Design review of the part built by this model. Coordinates are the model's own, in mm. A direction names the side the tool comes from. Give positions to 0.01 mm unless a question says otherwise; leave off trailing zeros. Loops run counter-clockwise (first coordinate to the right, second up) from the corner with the lowest first, then second, coordinate; pieces in that order, holes last. Notation, with made-up numbers: (58.5, 3.5) - (65.5, 3.5) arc R30 cw to (65.5, 33.5) - close; hole circle Ø10 at (33.25, 44). An arc over 180 degrees is marked (long way). Write each question's results on one line, items separated by ' | '.
```python
from build123d import *

# Parameters (mm, degrees)
SKETCH1_W           = 11
SKETCH1_H           = 12
BOSS_EXTRUDE1_DEPTH = 1.8
SKETCH2_W           = 2.54
SKETCH2_H           = 10.16
BOSS_EXTRUDE2_DEPTH = 2.54
BOSS_EXTRUDE3_START = -5.84
SKETCH3_W           = 0.5
SKETCH3_H           = 0.5
BOSS_EXTRUDE3_DEPTH = 12.34
SKETCH4_W           = 5.5
SKETCH4_H           = 4
BOSS_EXTRUDE4_DEPTH = 2
CHAMFER1_SIZE       = 0.5
SKETCH5_W           = 0.8
SKETCH5_H           = 7
BOSS_EXTRUDE5_DEPTH = 0.4
SKETCH6_R           = 0.5
CUT_EXTRUDE1_DEPTH  = 0.1
SKETCH7_R           = 0.25
CUT_EXTRUDE2_DEPTH  = 0.1


with BuildPart() as part:
    # Sketch1 → Boss-Extrude1 (new body)
    with BuildSketch(Plane(origin=(0, 0, 0), x_dir=(1, 0, 0), z_dir=(0, 1, 0))):
        Rectangle(SKETCH1_W, SKETCH1_H)
    extrude(amount=BOSS_EXTRUDE1_DEPTH)

    # Sketch2 → Boss-Extrude2 (add)
    with BuildSketch(Plane.XZ):
        with Locations((-3.81, 0)):
            Rectangle(SKETCH2_W, SKETCH2_H)
        with Locations((3.81, 0)):
            Rectangle(SKETCH2_W, SKETCH2_H)
    extrude(amount=BOSS_EXTRUDE2_DEPTH)

    # Sketch3 → Boss-Extrude3 (add)
    with BuildSketch(Plane.XZ.offset(2.54).offset(BOSS_EXTRUDE3_START)):
        with Locations((3.81, 1.27)):
            Rectangle(SKETCH3_W, SKETCH3_H)
        with Locations((3.81, 3.81)):
            Rectangle(SKETCH3_W, SKETCH3_H)
        with Locations((3.81, -1.27)):
            Rectangle(SKETCH3_W, SKETCH3_H)
        with Locations((3.81, -3.81)):
            Rectangle(SKETCH3_W, SKETCH3_H)
    boss_extrude3 = extrude(amount=BOSS_EXTRUDE3_DEPTH)

    # Mirror1: Boss-Extrude3 across plane
    add(boss_extrude3.mirror(Plane(origin=(0, 0, 0), x_dir=(0, 0, 1), z_dir=(1, 0, 0))))

    # Sketch4 → Boss-Extrude4 (add)
    with BuildSketch(Plane(origin=(0, 1.8, 0), x_dir=(1, 0, 0), z_dir=(0, 1, 0))):
        Rectangle(SKETCH4_W, SKETCH4_H)
    extrude(amount=BOSS_EXTRUDE4_DEPTH)

    # Chamfer1
    chamfer1_edges = [part.edges().sort_by_distance(p)[0] for p in [
        (0, 3.8, -2),
        (0, 3.8, 2),
    ]]
    chamfer(chamfer1_edges, length=CHAMFER1_SIZE)

    # Sketch5 → Boss-Extrude5 (add)
    with BuildSketch(Plane(origin=(0, 1.8, 0), x_dir=(1, 0, 0), z_dir=(0, 1, 0))):
        with Locations((-0.635, 0)):
            Rectangle(SKETCH5_W, SKETCH5_H)
        with Locations((-1.905, 0)):
            Rectangle(SKETCH5_W, SKETCH5_H)
        with Locations((0.635, 0)):
            Rectangle(SKETCH5_W, SKETCH5_H)
        with Locations((1.905, 0)):
            Rectangle(SKETCH5_W, SKETCH5_H)
    extrude(amount=BOSS_EXTRUDE5_DEPTH)

    # Sketch6 → Cut-Extrude1 (cut)
    with BuildSketch(Plane(origin=(0, 1.8, 0), x_dir=(1, 0, 0), z_dir=(0, 1, 0))):
        with Locations(Location((-3.81, 5.03, 0), (0, 0, 270))):
            Circle(SKETCH6_R)
    extrude(amount=-CUT_EXTRUDE1_DEPTH, mode=Mode.SUBTRACT)

    # Sketch7 → Cut-Extrude2 (cut)
    with BuildSketch(Plane(origin=(0, 3.8, 0), x_dir=(1, 0, 0), z_dir=(0, 1, 0))):
        with Locations(Location((-2.25, -1, 0), (0, 0, 270))):
            Circle(SKETCH7_R)
    extrude(amount=-CUT_EXTRUDE2_DEPTH, mode=Mode.SUBTRACT)


solid = part.part
```
Item 1: Clearance check with flat-ended pins moving along their axes: P1, Ø0.8, axis at x = 4.5, y = -1.5, coming from the -Z side; P2, Ø4, axis at x = 0, z = 3, coming from the +Y side; P3, Ø0.6, axis at y = 2.5, z = 4, coming from the -X side; P4, Ø0.6, axis at x = 3.5, y = 2.5, coming from the +Z side. State where each tip first meets the part, or that it passes through.
Output values:
P1: stops at z = -5.08 | P2: stops at y = 3.8 | P3: stops at x = -4.06 | P4: stops at z = 4.06
Item 2: We need section B-B on y = -6. Give the number of separate pieces and of enclosed holes in the cut face, then the cut area to 3 significant figures.
Output values:
separate pieces: 8 | enclosed holes: 0 | area: 2.00 mm²
Item 3: We need section A-A on y = -1.75. Give the boundary of the cut face in (x, z).
Output values:
outline: (-5.08, -5.08) - (-2.54, -5.08) - (-2.54, 5.08) - (-5.08, 5.08) - close; (2.54, -5.08) - (5.08, -5.08) - (5.08, 5.08) - (2.54, 5.08) - close
Item 4: Draft analysis for pull direction Z (two halves, no side actions). For faces 5 (the face through (4, -1, -5.08)), 6 (the face through (-5.5, 1, 0)), 7 (the face through (-4, 1.7, -5)), 8 (the face through (0, 1, 6)), state which applies: +Z half, -Z half, draft (parallel to the pull), parting line (faces both ways), or undercut.
Output values:
face 5: -Z half | face 6: draft | face 7: undercut | face 8: +Z half
Item 5: We need section D-D on x = -0.5. Give the boundary of the cut face in (y, z), then the cut area to 4 significant figures.
Output values:
outline: (0, -6) - (1.8, -6) - (1.8, -3.5) - (2.2, -3.5) - (2.2, -2) - (3.3, -2) - (3.8, -1.5) - (3.8, 1.5) - (3.3, 2) - (2.2, 2) - (2.2, 3.5) - (1.8, 3.5) - (1.8, 6) - (0, 6) - close | area: 30.55 mm²
Item 6: We need section C-C on z = 0. Give the boundary of the cut face in (x, y).
Output values:
outline: (-5.5, 0) - (-5.08, 0) - (-5.08, -2.54) - (-2.54, -2.54) - (-2.54, 0) - (2.54, 0) - (2.54, -2.54) - (5.08, -2.54) - (5.08, 0) - (5.5, 0) - (5.5, 1.8) - (2.75, 1.8) - (2.75, 3.8) - (-2.75, 3.8) - (-2.75, 1.8) - (-5.5, 1.8) - close
Item 7: Tool access review of faces 1 (the face through (-5.08, -1, 0)), 2 (the face through (-2, 2.2, 3)), 3 (the face through (2, 2.2, -3)), 4 (the face through (-2.75, 3, 0)): name each direction out of +Z, -Z, +X, -X, +Y, -Y from which nothing blocks a thin tool from reaching the whole face with its end or side.
Output values:
face 1: +Z, -Z, -X, -Y | face 2: +Z, +X, -X, +Y | face 3: -Z, +X, -X, +Y | face 4: +Z, -Z, +Y
Item 8: Wall thickness on probe 1 along X at (y, z) = (-0.5, -2.25); probe 2 along Y at (x, z) = (-2.25, -4.5); probe 3 along Z at (x, y) = (-4.75, -2.5): over which ranges is each line inside the solid? List them lowest first.
Output values:
probe 1: x = -5.08 to -2.54, 2.54 to 5.08 | probe 2: y = 0 to 1.8 | probe 3: z = -5.08 to 5.08
